from build123d import *

# Parameters (mm, degrees)
BOSS_EXTRUDE1_DEPTH     = 50
SKETCH2_W               = 360
SKETCH2_H               = 25
BOSS_EXTRUDE3_DEPTH     = 230
SKETCH3_W               = 260
SKETCH3_H               = 130
CUT_EXTRUDE1_DEPTH      = 230
BOSS_EXTRUDE4_DEPTH     = 1250
BOSS_EXTRUDE5_DEPTH     = 1250
SKETCH7_W               = 46
SKETCH7_H               = 50
BOSS_EXTRUDE6_DEPTH     = 700
SKETCH10_W              = 50
SKETCH10_H              = 25
BOSS_EXTRUDE7_DEPTH     = 992
SKETCH11_R              = 7.5
CUT_EXTRUDE2_DEPTH      = 1012
SKETCH12_W              = 50
SKETCH12_H              = 50
BOSS_EXTRUDE8_DEPTH     = 4
SKETCH13_W              = 4
SKETCH13_H              = 50
BOSS_EXTRUDE9_DEPTH     = 50
SKETCH15_R              = 7.5
CUT_EXTRUDE3_DEPTH      = 380
CUT_EXTRUDE5_DEPTH      = 1743.470523401
CUT_EXTRUDE5_DEPTH_BACK = 1743.470523401
SKETCH16_R              = 7.5
SKETCH17_W              = 25
SKETCH17_H              = 50
BOSS_EXTRUDE10_DEPTH    = 250
SKETCH18_R              = 7.5
CUT_EXTRUDE6_DEPTH      = 250


with BuildPart() as part:
    # Sketch1 → Boss-Extrude1 (new body)
    with BuildSketch(Plane.XY):
        Polygon((-915.830763168, 0), (34.169236832, 0), (34.169236832, 155), (59.169236832, 155), (59.169236832, -25), (-940.830763168, -25), (-940.830763168, 155), (-915.830763168, 155), align=None)
    extrude(amount=-BOSS_EXTRUDE1_DEPTH)

    # Sketch2 → Boss-Extrude3 (add)
    with BuildSketch(Plane.XY):
        with Locations((-440.830763168, -12.5)):
            Rectangle(SKETCH2_W, SKETCH2_H)
    extrude(amount=-BOSS_EXTRUDE3_DEPTH)

    # Sketch3 → Cut-Extrude1 (cut)
    with BuildSketch(Plane(origin=(0, 0, 0), x_dir=(1, 0, 0), z_dir=(0, 1, 0))):
        with Locations((-440.830763168, 115)):
            Rectangle(SKETCH3_W, SKETCH3_H)
    extrude(amount=-CUT_EXTRUDE1_DEPTH, mode=Mode.SUBTRACT)

    # Sketch4 → Boss-Extrude4 (add)
    with BuildSketch(Plane(origin=(0, 0, -50), x_dir=(-1, 0, 0), z_dir=(0, 0, -1))):
        Polygon((-59.169236832, 25), (-59.169236832, -25), (-9.169236832, -25), (-9.169236832, -21), (-55.169236832, -21), (-55.169236832, 25), align=None)
    extrude(amount=BOSS_EXTRUDE4_DEPTH)

    # Sketch6 → Boss-Extrude5 (add)
    with BuildSketch(Plane(origin=(0, 0, -50), x_dir=(-1, 0, 0), z_dir=(0, 0, -1))):
        Polygon((940.830763168, 25), (940.830763168, -25), (890.830763168, -25), (890.830763168, -21), (936.830763168, -21), (936.830763168, 25), align=None)
    extrude(amount=BOSS_EXTRUDE5_DEPTH)

    # Sketch7 → Boss-Extrude6 (add)
    with BuildSketch(Plane(origin=(0, -21, 0), x_dir=(1, 0, 0), z_dir=(0, 1, 0))):
        with Locations((-913.830763168, 1265.818413322)):
            Rectangle(SKETCH7_W, SKETCH7_H)
        with Locations((32.169236832, 1265.818413322)):
            Rectangle(SKETCH7_W, SKETCH7_H)
    extrude(amount=BOSS_EXTRUDE6_DEPTH)

    # Sketch10 → Boss-Extrude7 (add)
    with BuildSketch(Plane(origin=(-936.830763168, 0, 0), x_dir=(0, 0, -1), z_dir=(1, 0, 0))):
        with Locations((1215.818413322, -8.5)):
            Rectangle(SKETCH10_W, SKETCH10_H)
    extrude(amount=BOSS_EXTRUDE7_DEPTH)

    # Sketch11 → Cut-Extrude2 (cut)
    with BuildSketch(Plane.ZY.offset(940.830763168)):
        with Locations((-25, 130)):
            Circle(SKETCH11_R)
    extrude(amount=-CUT_EXTRUDE2_DEPTH, mode=Mode.SUBTRACT)

    # Sketch12 → Boss-Extrude8 (add)
    with BuildSketch(Plane(origin=(0, 0, 0), x_dir=(1, 0, 0), z_dir=(0, 1, 0))):
        with Locations((-575.830763168, 204.911627509)):
            Rectangle(SKETCH12_W, SKETCH12_H)
        with Locations((-305.830763168, 204.911627509)):
            Rectangle(SKETCH12_W, SKETCH12_H)
    extrude(amount=BOSS_EXTRUDE8_DEPTH)

    # Sketch13 → Boss-Extrude9 (add)
    with BuildSketch(Plane(origin=(0, 0, 0), x_dir=(1, 0, 0), z_dir=(0, 1, 0))):
        with Locations((-598.830763168, 204.911627509)):
            Rectangle(SKETCH13_W, SKETCH13_H)
        with Locations((-278.830763168, 204.911627509)):
            Rectangle(SKETCH13_W, SKETCH13_H)
    extrude(amount=BOSS_EXTRUDE9_DEPTH)

    # Sketch15 → Cut-Extrude3 (cut)
    with BuildSketch(Plane.ZY.offset(600.830763168)):
        with Locations((-204.911627509, 40)):
            Circle(SKETCH15_R)
    extrude(amount=-CUT_EXTRUDE3_DEPTH, mode=Mode.SUBTRACT)

    # Sketch16 → Cut-Extrude5 (cut, two sides: drawn at the far end of the back side and taken through both)
    with BuildSketch(Plane(origin=(0, 0, 0), x_dir=(0, 0, -1), z_dir=(1, 0, 0)).offset(-CUT_EXTRUDE5_DEPTH_BACK)):
        with Locations((1268.318413322, 604)):
            Circle(SKETCH16_R)
    extrude(amount=CUT_EXTRUDE5_DEPTH + CUT_EXTRUDE5_DEPTH_BACK, mode=Mode.SUBTRACT)

    # Sketch17 → Boss-Extrude10 (add)
    with BuildSketch(Plane(origin=(0, 4, 0), x_dir=(1, 0, 0), z_dir=(0, 1, 0))):
        with Locations((-508.330763168, 1215.818413322)):
            Rectangle(SKETCH17_W, SKETCH17_H)
        with Locations((-373.330763168, 1215.818413322)):
            Rectangle(SKETCH17_W, SKETCH17_H)
    extrude(amount=BOSS_EXTRUDE10_DEPTH)

    # Sketch18 → Cut-Extrude6 (cut)
    with BuildSketch(Plane.ZY.offset(520.830763168)):
        with Locations((-1214.592207536, 214)):
            Circle(SKETCH18_R)
    extrude(amount=-CUT_EXTRUDE6_DEPTH, mode=Mode.SUBTRACT)


solid = part.part
Verification items for the finished model (mm, model axes). A direction names the side the tool comes from. Round coordinates to 2 decimals unless told otherwise and drop trailing zeros. Loops run counter-clockwise (first coordinate to the right, second up) from the corner with the lowest first, then second, coordinate; pieces in that order, holes last. Notation, with made-up numbers: (35.25, 47) - (70.25, 47) arc R30 ccw to (70.25, 71) - close; hole circle Ø9 at (64.25, -6.75). An arc over 180 degrees is marked (long way). Use a Markdown table: item, result. Add a question column.
1. Section check C-C, the plane z = -133.5. Record the boundary of the cut face in (x, y), plus the area to 3 significant figures.
2. Section check D-D, the plane x = -10. Record the boundary of the cut face in (y, z), plus the area to 3 significant figures.
3. Section check B-B, the plane y = 481. Record the boundary of the cut face in (x, z), plus the area to 3 significant figures.
4. Gauge pin test, flat ends, axial feed: pin 1 (12.5 mm diameter, centred on x = 51.5, z = -28.5, fed in from +Y); pin 2 (10 mm diameter, centred on x = 42, z = -1296.5, fed in from +Y); pin 3 (15 mm diameter, centred on y = 328, z = -1253.5, fed in from +X); pin 4 (12 mm diameter, centred on y = 40, z = -204.91, fed in from -X). Record the tip position at first contact, or that the pin passes through.
5. Thickness scan on probe 1 along Y at (x, z) = (-934, -25). Record the ranges inside material, lowest first. Write a range as [from, to].
6. Access from +Z, -Z, +X, -X, +Y, -Y to the whole of each face (thin tool, end or side, straight path). Record for faces 1 (the face through (-442.9, 3.8, -1240.818)), 2 (the face through (-936.831, 347, -1265)), 3 (the face through (32, -21, -612)), 4 (the face through (34.169, 76, -25)).
7. Release check for a two-part mould opening along Z. For faces 5 (the face through (-495.831, 127, -1215)), 6 (the face through (-938, -11, -1300)), 7 (the face through (-292, 3, -229.912)) record: released by +Z, released by -Z, zero draft, split by the parting line, or undercut.
8. Section check A-A, the plane x = -457. Record the boundary of the cut face in (y, z).
Checks:
| question | item | result |
|---|---|---|
| 1 | outline | (-940.83, -25) - (-890.83, -25) - (-890.83, -21) - (-936.83, -21) - (-936.83, 25) - (-940.83, 25) - close; (-620.83, -25) - (-570.83, -25) - (-570.83, 0) - (-620.83, 0) - close; (-310.83, -25) - (-260.83, -25) - (-260.83, 0) - (-310.83, 0) - close; (9.17, -25) - (59.17, -25) - (59.17, 25) - (55.17, 25) - (55.17, -21) - (9.17, -21) - close |
| 1 | area | 3,270 mm^2 |
| 2 | outline | (-25, -50) - (0, -50) - (0, 0) - (-25, 0) - close; (-21, -1240.82) - (4, -1240.82) - (4, -1190.82) - (-21, -1190.82) - close |
| 2 | area | 2,500 mm^2 |
| 3 | outline | (-936.83, -1290.82) - (-890.83, -1290.82) - (-890.83, -1240.82) - (-936.83, -1240.82) - close; (9.17, -1290.82) - (55.17, -1290.82) - (55.17, -1240.82) - (9.17, -1240.82) - close |
| 3 | area | 4,600 mm^2 |
| 4 | pin 1 | stops at y = 155 |
| 4 | pin 2 | stops at y = -21 |
| 4 | pin 3 | stops at x = 55.17 |
| 4 | pin 4 | passes through |
| 5 | probe 1 | y = [-25, 122.5], [137.5, 155] |
| 6 | face 1 | -Z, +Y, -Y |
| 6 | face 2 | -Z, -X, +Y |
| 6 | face 3 | +Y |
| 6 | face 4 | +Z, +Y |
| 7 | face 5 | zero draft |
| 7 | face 6 | released by -Z |
| 7 | face 7 | undercut |
| 8 | outline | (-25, -230) - (0, -230) - (0, -180) - (-25, -180) - close; (-25, -50) - (0, -50) - (0, 0) - (-25, 0) - close; (-21, -1240.82) - (4, -1240.82) - (4, -1190.82) - (-21, -1190.82) - close |
